CAD build for the part. Positions are in the model's coordinates, mm. Face numbers are marked on the shaded views. Round coordinates to 2 decimals unless told otherwise and drop trailing zeros. Order: outer loops, then holes, each group sorted by start corner. A loop starts at its lowest first (then second) coordinate and runs counter-clockwise, first axis right, second up. Notation, with made-up numbers: M 72,-2.75 L 131,-2.75 A17 ccw 131,6.25 Z; hole C -16,6 d11. An arc over 180 degrees is marked long. Answer as a JSON object with one key per item and string values. Group by question number.
```python
from build123d import *

# Parameters (mm, degrees)
ESQUISSE1_R             = 10
BOSS_EXTRU_1_DEPTH      = 15
ESQUISSE2_R             = 9.5
ESQUISSE2_R_2           = 3.85
ENL_V_MAT_EXTRU_1_DEPTH = 0.5
ESQUISSE3_R             = 0.75
BOSS_EXTRU_2_DEPTH      = 3
CONG_1_R                = 0.5
ESQUISSE4_W             = 28
ESQUISSE4_H             = 40
BOSS_EXTRU_3_DEPTH      = 1
ESQUISSE5_W             = 10
ESQUISSE5_H             = 2
BOSS_EXTRU_4_DEPTH      = 2
ESQUISSE6_W             = 1
ESQUISSE6_H             = 1
BOSS_EXTRU_5_DEPTH      = 2
ESQUISSE8_W             = 1
ESQUISSE8_H             = 1
BOSS_EXTRU_6_DEPTH      = 5


with BuildPart() as part:
    # Esquisse1 → Boss.-Extru.1 (new body)
    with BuildSketch(Plane(origin=(0, 0, 0), x_dir=(1, 0, 0), z_dir=(0, 1, 0))):
        with Locations(Location((0, 0, 0), (0, 0, 270))):
            Circle(ESQUISSE1_R)
    extrude(amount=BOSS_EXTRU_1_DEPTH)

    # Esquisse2 → Enlèv. mat.-Extru.1 (cut)
    with BuildSketch(Plane(origin=(0, 15, 0), x_dir=(1, 0, 0), z_dir=(0, 1, 0))):
        with Locations(Location((0, 0, 0), (0, 0, 270))):
            Circle(ESQUISSE2_R)
        with Locations(Location((0, 0, 0), (0, 0, 270))):
            Circle(ESQUISSE2_R_2, mode=Mode.SUBTRACT)
    extrude(amount=-ENL_V_MAT_EXTRU_1_DEPTH, mode=Mode.SUBTRACT)

    # Esquisse3 → Boss.-Extru.2 (add)
    with BuildSketch(Plane.XY.offset(9)):
        with Locations(Location((0, 1.513817118, 0), (0, 0, 180))):
            Circle(ESQUISSE3_R)
    extrude(amount=BOSS_EXTRU_2_DEPTH)

    # Congé1
    cong_1_edges = [part.edges().sort_by_distance(p)[0] for p in [
        (0.75, 1.513817118, 9.971835338),
    ]]
    fillet(cong_1_edges, radius=CONG_1_R)

    # Esquisse4 → Boss.-Extru.3 (add)
    with BuildSketch(Plane.XZ):
        with Locations((0.33364204, 9.631825749)):
            Rectangle(ESQUISSE4_W, ESQUISSE4_H)
    extrude(amount=BOSS_EXTRU_3_DEPTH)

    # Esquisse5 → Boss.-Extru.4 (add)
    with BuildSketch(Plane(origin=(0, 0, 0), x_dir=(1, 0, 0), z_dir=(0, 1, 0))):
        with Locations((0.33364204, -25.631825749)):
            Rectangle(ESQUISSE5_W, ESQUISSE5_H)
    extrude(amount=BOSS_EXTRU_4_DEPTH)

    # Esquisse6 → Boss.-Extru.5 (add)
    with BuildSketch(Plane(origin=(0, 2, 0), x_dir=(1, 0, 0), z_dir=(0, 1, 0))):
        with Locations((-2.66635796, -25.631825749)):
            Rectangle(ESQUISSE6_W, ESQUISSE6_H)
        with Locations((0.33364204, -25.631825749)):
            Rectangle(ESQUISSE6_W, ESQUISSE6_H)
        with Locations((3.33364204, -25.631825749)):
            Rectangle(ESQUISSE6_W, ESQUISSE6_H)
    extrude(amount=BOSS_EXTRU_5_DEPTH)

    # Esquisse8 → Boss.-Extru.6 (add)
    with BuildSketch(Plane.XY.offset(26.131825749)):
        with Locations((-2.66635796, 3.5)):
            Rectangle(ESQUISSE8_W, ESQUISSE8_H)
        with Locations((0.33364204, 3.5)):
            Rectangle(ESQUISSE8_W, ESQUISSE8_H)
        with Locations((3.33364204, 3.5)):
            Rectangle(ESQUISSE8_W, ESQUISSE8_H)
    extrude(amount=BOSS_EXTRU_6_DEPTH)


solid = part.part
```
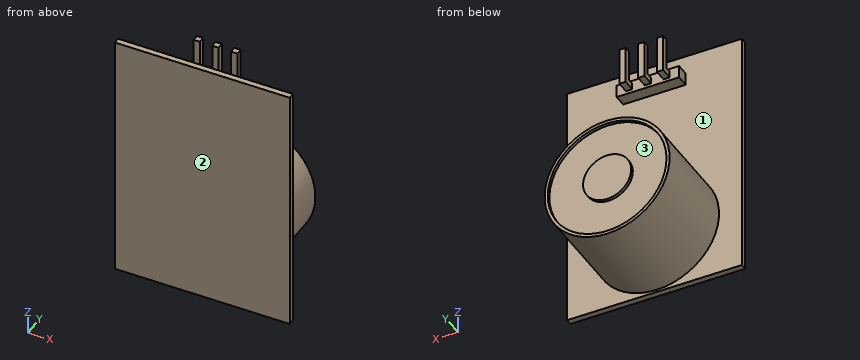
Item 1: Cut at B-B, the plane x = -6.5. Give the cut face in (y, z), and give its area (3 significant figures).
Item 2: Flat gauge pins, fed straight in: pin 1 Ø1.6 at (y, z) = (3.5, 28.5) entering from -X; pin 2 Ø1.6 at (y, z) = (3.5, 27) entering from +X; pin 3 Ø12 at (x, z) = (3.5, -2.5) entering from +Y; pin 4 Ø0.8 at (x, y) = (-3, 3) entering from -Z. Where does each tip first touch, or does it go through?
Item 3: Cut at C-C, the plane y = 5. Give the cut face in (x, z).
Item 4: Cut at A-A, the plane z = 0. Give the cut face in (x, y).
Item 5: Cut at D-D, the plane z = 4.5. Give the cut face in (x, y).
Item 6: Two-plate mould, pull along Z, no slides. Class the marked faces 1, 2 and 3: +Z half, -Z half, draft (parallel to the pull), parting line (faces both ways), or undercut.
Item 7: Drill centre lines: line 1 (X direction, y = 14.7, z = 0); line 2 (Y direction, x = -0.5, z = 4.5); line 3 (Y direction, x = -11.75, z = -7.5). Where is each one in solid material? Low to high. Write a range as [from, to].
Response values:
{
 "1": {"outline": "M -1,-10.37 L 0,-10.37 L 0,-7.6 L 15,-7.6 L 15,-6.93 L 14.5,-6.93 L 14.5,6.93 L 15,6.93 L 15,7.6 L 0,7.6 L 0,29.63 L -1,29.63 Z", "area": "261 mm^2"},
 "2": {"pin 1": "x = -3.17", "pin 2": "x = 3.83", "pin 3": "y = 15", "pin 4": "z = -9.66"},
 "3": {"outline": "C 0,0 d20"},
 "4": {"outline": "M -13.67,-1 L 14.33,-1 L 14.33,0 L 10,0 L 10,15 L 9.5,15 L 9.5,14.5 L 3.85,14.5 L 3.85,15 L -3.85,15 L -3.85,14.5 L -9.5,14.5 L -9.5,15 L -10,15 L -10,0 L -13.67,0 Z"},
 "5": {"outline": "M -13.67,-1 L 14.33,-1 L 14.33,0 L 8.93,0 L 8.93,15 L 8.37,15 L 8.37,14.5 L -8.37,14.5 L -8.37,15 L -8.93,15 L -8.93,0 L -13.67,0 Z"},
 "6": {"face 1": "undercut", "face 2": "draft", "face 3": "undercut"},
 "7": {"line 1": "[-10, -9.5], [-3.85, 3.85], [9.5, 10]", "line 2": "[-1, 14.5]", "line 3": "[-1, 0]"}
}
